```python
from build123d import *

# Parameters (mm, degrees)
SKETCH_1_R          = 6
SKETCH_1_R_2        = 4
EXTRUDE_1_DEPTH     = 4
SKETCH_2_R          = 6.8
SKETCH_2_R_2        = 6
EXTRUDE_2_DEPTH     = 0.8
SKETCH_3_R          = 5.5
SKETCH_3_R_2        = 4.5
CUT_EXTRUDE_1_DEPTH = 0.2


with BuildPart() as part:
    # 草图1 → 凸台-拉伸1 (new body)
    with BuildSketch(Plane(origin=(0, 0, 0), x_dir=(1, 0, 0), z_dir=(0, 1, 0))):
        with Locations(Location((0, 0, 0), (0, 0, 270))):
            Circle(SKETCH_1_R)
        with Locations(Location((0, 0, 0), (0, 0, 270))):
            Circle(SKETCH_1_R_2, mode=Mode.SUBTRACT)
    extrude(amount=EXTRUDE_1_DEPTH)

    # 草图2 → 凸台-拉伸2 (add)
    with BuildSketch(Plane(origin=(0, 0, 0), x_dir=(1, 0, 0), z_dir=(0, 1, 0))):
        with Locations(Location((0, 0, 0), (0, 0, 270))):
            Circle(SKETCH_2_R)
        with Locations(Location((0, 0, 0), (0, 0, 270))):
            Circle(SKETCH_2_R_2, mode=Mode.SUBTRACT)
    extrude(amount=EXTRUDE_2_DEPTH)

    # 草图3 → 切除-拉伸1 (cut)
    with BuildSketch(Plane(origin=(0, 4, 0), x_dir=(1, 0, 0), z_dir=(0, 1, 0))):
        with Locations(Location((0, 0, 0), (0, 0, 270))):
            Circle(SKETCH_3_R)
        with Locations(Location((0, 0, 0), (0, 0, 270))):
            Circle(SKETCH_3_R_2, mode=Mode.SUBTRACT)
    cut_extrude_1 = extrude(amount=-CUT_EXTRUDE_1_DEPTH, mode=Mode.SUBTRACT)

    # 镜向1: 切除-拉伸1 across plane
    add(cut_extrude_1.mirror(Plane.ZX.offset(2)), mode=Mode.SUBTRACT)


solid = part.part
```
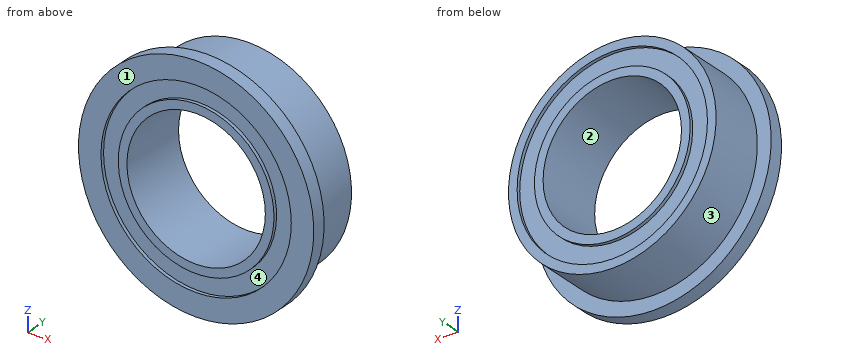
Input: part model. Units: mm. Frame: model coordinates. Face numbers are marked on the shaded views. Coordinates: 2 decimals unless noted, no trailing zeros. Write each loop counter-clockwise with the first axis right and the second up, starting at its lowest first coordinate (ties: lowest second). Pieces come first, ordered by that corner, then holes. Notation, with made-up numbers: (-17, 16.5) -> (-11, 16.5) arc R16 cw to (-11, 20.5) -> close; hole circle Ø2 at (55, 13). An arc over 180 degrees is marked (long way). Write each question's results on one line, items separated by ' | '.
Item 1: Section query D-D on z = 5.25. Return loops of the section in (x, y).
Conclusion:
outline: (-4.32, 0) -> (-1.64, 0) -> (-1.64, 0.2) -> (1.64, 0.2) -> (1.64, 0) -> (4.32, 0) -> (4.32, 0.8) -> (2.9, 0.8) -> (2.9, 4) -> (1.64, 4) -> (1.64, 3.8) -> (-1.64, 3.8) -> (-1.64, 4) -> (-2.9, 4) -> (-2.9, 0.8) -> (-4.32, 0.8) -> close
Item 2: Mould query, pull axis X, two halves, no side actions, for the marked faces 1, 2, 3 and 4. Classes: +X half, -X half, draft (parallel to the pull), parting line (faces both ways), or undercut.
Conclusion:
face 1: draft | face 2: undercut | face 3: parting line | face 4: undercut
Item 3: Material intervals for probe 1 along X at (y, z) = (3.9, 0); probe 2 along X at (y, z) = (0.15, 0); probe 3 along X at (y, z) = (2, 0), sorted ascending.
Conclusion:
probe 1: x = -6 to -5.5, -4.5 to -4, 4 to 4.5, 5.5 to 6 | probe 2: x = -6.8 to -5.5, -4.5 to -4, 4 to 4.5, 5.5 to 6.8 | probe 3: x = -6 to -4, 4 to 6
Item 4: Section query C-C on y = 2.8. Return loops of the section in (x, z), plus the area to 3 significant figures.
Conclusion:
outline: circle Ø12 at (0, 0); hole circle Ø8 at (0, 0) | area: 62.8 mm^2
Item 5: Section query A-A on z = 0. Return loops of the section in (x, y), plus the area to 3 significant figures.
Conclusion:
outline: (-6.8, 0) -> (-5.5, 0) -> (-5.5, 0.2) -> (-4.5, 0.2) -> (-4.5, 0) -> (-4, 0) -> (-4, 4) -> (-4.5, 4) -> (-4.5, 3.8) -> (-5.5, 3.8) -> (-5.5, 4) -> (-6, 4) -> (-6, 0.8) -> (-6.8, 0.8) -> close; (4, 0) -> (4.5, 0) -> (4.5, 0.2) -> (5.5, 0.2) -> (5.5, 0) -> (6.8, 0) -> (6.8, 0.8) -> (6, 0.8) -> (6, 4) -> (5.5, 4) -> (5.5, 3.8) -> (4.5, 3.8) -> (4.5, 4) -> (4, 4) -> close | area: 16.5 mm^2
Item 6: Section query B-B on x = 0. Return loops of the section in (y, z), plus the area to 3 significant figures.
Conclusion:
outline: (0, -6.8) -> (0.8, -6.8) -> (0.8, -6) -> (4, -6) -> (4, -5.5) -> (3.8, -5.5) -> (3.8, -4.5) -> (4, -4.5) -> (4, -4) -> (0, -4) -> (0, -4.5) -> (0.2, -4.5) -> (0.2, -5.5) -> (0, -5.5) -> close; (0, 4) -> (4, 4) -> (4, 4.5) -> (3.8, 4.5) -> (3.8, 5.5) -> (4, 5.5) -> (4, 6) -> (0.8, 6) -> (0.8, 6.8) -> (0, 6.8) -> (0, 5.5) -> (0.2, 5.5) -> (0.2, 4.5) -> (0, 4.5) -> close | area: 16.5 mm^2
Item 7: Pin query (flat end, axial travel): pin 1 Ø1.5 at (x, y) = (-5.5, 1) entering from -Z; pin 2 Ø1 at (y, z) = (3.5, -2) entering from -X; pin 3 Ø1.5 at (x, y) = (4.5, 1) entering from +Z. Return the tip coordinate at first contact, or that it passes through.
Conclusion:
pin 1: stops at z = -4.84 | pin 2: stops at x = -5.81 | pin 3: stops at z = 5.65
